Design review of the part built by this model. Coordinates are the model's own, in mm. Coordinates: 2 decimals unless noted, no trailing zeros. Write each loop counter-clockwise with the first axis right and the second up, starting at its lowest first coordinate (ties: lowest second). Pieces come first, ordered by that corner, then holes. Notation, with made-up numbers: M -33,-18 L 19,-18 A34 ccw 19,12 Z; hole C 76,18 d3. An arc over 180 degrees is marked long. Write each question's results on one line, items separated by ' | '. Start each with the question number.
```python
from build123d import *

# Parameters (mm, degrees)
F0_W     = 60
F0_H     = 37
F0_R     = 1.55
F0_R_2   = 4
F1_DEPTH = 3


with BuildPart() as f1:
    # F0 (on Front) → F1 (new body)
    with BuildSketch(Plane.XZ):
        with Locations((17, 5)):
            Rectangle(F0_W, F0_H)
        with Locations((-8, 0)):
            Circle(F0_R, mode=Mode.SUBTRACT)
        Circle(F0_R_2, mode=Mode.SUBTRACT)
        with Locations((8, 0)):
            Circle(F0_R, mode=Mode.SUBTRACT)
    extrude(amount=F1_DEPTH)


solid = f1.part
```
Item 1: Draft analysis for pull direction Z (two halves, no side actions). For faces 1 (the cylindrical face through (-6.522, -1.479, 0.466)), 2 (the flat face through (17, -1, 23.5)), 3 (the flat face through (17, -3, 5)), state which applies: released by +Z, released by -Z, zero draft, split by the parting line, or undercut.
Item 2: We need section D-D on x = 0. State the section outline as (y, z) points.
Item 3: We need section C-C on z = 0. State the section outline as (x, y) points.
Item 4: We need section A-A on x = 8. State the section outline as (y, z) points, then the cut area to 3 significant figures.
Item 5: Wall thickness on L1, parallel to Z at x = -8, y = -1.65; L2, parallel to Z at x = 0, y = -0.9; L3, parallel to X at y = -2.25, z = 0.5: over which ranges is each line inside the solid? List them lowest first.
Item 6: Insertion check: pin 1 Ø3 at (x, z) = (-8, 0) entering from -Y; pin 2 Ø8 at (x, z) = (-3.5, 14) entering from +Y. Each pin has a flat end and moves straight along its axis. Give the tip position at first contact, or say it passes through.
Item 7: We need section B-B on y = -0.5. State the section outline as (x, z) points, then the cut area to 3 significant figures.
Answer:
1) face 1: undercut | face 2: released by +Z | face 3: zero draft
2) outline: M -3,-13.5 L 0,-13.5 L 0,-4 L -3,-4 Z; M -3,4 L 0,4 L 0,23.5 L -3,23.5 Z
3) outline: M -13,-3 L -9.55,-3 L -9.55,0 L -13,0 Z; M -6.45,-3 L -4,-3 L -4,0 L -6.45,0 Z; M 4,-3 L 6.45,-3 L 6.45,0 L 4,0 Z; M 9.55,-3 L 47,-3 L 47,0 L 9.55,0 Z
4) outline: M -3,-13.5 L 0,-13.5 L 0,-1.55 L -3,-1.55 Z; M -3,1.55 L 0,1.55 L 0,23.5 L -3,23.5 Z | area: 102 mm^2
5) L1: z = -13.5 to -1.55, 1.55 to 23.5 | L2: z = -13.5 to -4, 4 to 23.5 | L3: x = -13 to -9.47, -6.53 to -3.97, 3.97 to 6.53, 9.47 to 47
6) pin 1: passes through | pin 2: stops at y = 0
7) outline: M -13,-13.5 L 47,-13.5 L 47,23.5 L -13,23.5 Z; hole C -8,0 d3.1; hole C 0,0 d8; hole C 8,0 d3.1 | area: 2,150 mm^2
